```python
from build123d import *

# Parameters (mm, degrees)
F1_DEPTH    = 6.35
F4_T1_DEPTH = 6.35
F2_W        = 2.032
F2_H        = 2.032
F5_DEPTH    = 0.508
F7_R        = 0.1905
F12_DEPTH   = 0.254


# Not quite as in the source:
# - a fillet or chamfer that OpenCascade refuses, or shapes differently, is made with other operations: its cross-section is extruded or revolved along the edge and cut away or added


with BuildPart() as f1:
    # F0 (on Front) → F1 (new body)
    with BuildSketch(Plane.XZ):
        with BuildLine():
            Line((0, 0.7623671392), (0, 0))
            Line((0, 0), (9.652, 0))
            Line((9.652, 0), (9.652, 0.7623671392))
            Line((9.652, 0.7623671392), (6.0225553446, 1.5280881198))
            Line((6.0225553446, 1.5280881198), (6.0735776823, 1.729142969))
            Line((6.0735776823, 1.729142969), (5.8725685775, 1.7715508037))
            Line((5.8725685775, 1.7715508037), (5.8107842668, 1.5280881198))
            ThreePointArc((5.8107842668, 1.5280881198), (4.826, 0.762), (3.8412157332, 1.5280881198))
            Line((3.8412157332, 1.5280881198), (3.7794314225, 1.7715508037))
            Line((3.7794314225, 1.7715508037), (3.5784223177, 1.729142969))
            Line((3.5784223177, 1.729142969), (3.6294446554, 1.5280881198))
            Line((3.6294446554, 1.5280881198), (0, 0.7623671392))
        make_face()
    extrude(amount=-F1_DEPTH)

    # F4: fillet of radius 0.254 on 2 edges, made by hand

    # F4_s2 → F4_t1 (join)
    with BuildSketch(Plane.XZ.offset(-6.35)):
        with BuildLine():
            ThreePointArc((6.2750780534, 1.4748122183), (6.1284229129, 1.5656081597), (6.0735776823, 1.729142969))
            Line((6.0735776823, 1.729142969), (6.0225553446, 1.5280881198))
            Line((6.0225553446, 1.5280881198), (6.2750780534, 1.4748122183))
        make_face()
        with BuildLine():
            ThreePointArc((3.5784223177, 1.729142969), (3.5235770871, 1.5656081597), (3.3769219466, 1.4748122183))
            Line((3.3769219466, 1.4748122183), (3.6294446554, 1.5280881198))
            Line((3.6294446554, 1.5280881198), (3.5784223177, 1.729142969))
        make_face()
    extrude(amount=F4_T1_DEPTH)

    # F2 (on face) → F5 (join)
    with BuildSketch(Plane(origin=(0.5652924546, 0, 2.6794324958), x_dir=(0.9784612522, 0, -0.2064305646), z_dir=(0.2064305646, 0, 0.9784612522))):
        with Locations((7.3553929503, 3.175)):
            Rectangle(F2_W, F2_H)
    f5 = extrude(amount=F5_DEPTH)

    # F6: F5 across plane
    add(f5.mirror(Plane.YZ.offset(4.826)))

    # F7
    f7_edges = [f1.edges().sort_by_distance(p)[0] for p in [
        (9.652, 3.175, 0.762367),
        (0, 3.175, 0.762367),
        (7.963539, 6.35, 1.11859),
        (7.963539, 0, 1.11859),
        (1.688461, 0, 1.11859),
        (1.688461, 6.35, 1.11859),
        (9.652, 0, 0.381184),
        (9.652, 6.35, 0.381184),
        (0, 0, 0.381184),
        (0, 6.35, 0.381184),
        (3.523577, 6.35, 1.565608),
        (3.523577, 0, 1.565608),
        (6.128423, 0, 1.565608),
        (6.128423, 6.35, 1.565608),
    ]]
    fillet(f7_edges, radius=F7_R)


with BuildPart() as f8_1:
    # F8: copy of F1
    add(f1.part)


with BuildPart() as f9_1:
    # F9: copy of F8_1
    add(f8_1.part)


with BuildPart() as f1_1:
    add(f1.part)

    # F12 (add): a face of the model
    f12_faces = [f1_1.faces().sort_by_distance(p)[0] for p in [
        (4.826, 3.175, 0),
    ]]
    extrude(f12_faces, amount=F12_DEPTH)


solid = f1_1.part
```
The model under review builds one solid part; all positions refer to its coordinate system, in mm. A direction names the side the tool comes from. Round coordinates to 2 decimals unless told otherwise and drop trailing zeros. Order: outer loops, then holes, each group sorted by start corner. A loop starts at its lowest first (then second) coordinate and runs counter-clockwise, first axis right, second up. Notation, with made-up numbers: M 5.25,-17.5 L 19.25,-17.5 A26 cw 19.25,4.5 Z; hole C 45,54 d6. An arc over 180 degrees is marked long. Use a Markdown table: item, result.
1) Draft analysis for pull direction Z (two halves, no side actions). For faces 1 (the face through (9.652, 3, 0)), 2 (the face through (4.845, 3.131, 0.762)), 3 (the face through (5, 3, -0.254)), state which applies: released by +Z, released by -Z, zero draft, split by the parting line, or undercut.
Report:
| item | result |
|---|---|
| face 1 | zero draft |
| face 2 | released by +Z |
| face 3 | released by -Z |
2) Insertion check: pin 1 (1 mm diameter, centred on y = 2.5, z = 1.5, fed in from -X); pin 2 (0.5 mm diameter, centred on x = 8, z = 1.5, fed in from +Y); pin 3 (0.7 mm diameter, centred on x = 8, z = 1.5, fed in from -Y). Each pin has a flat end and moves straight along its axis. Give the tip position at first contact, or say it passes through.
Report:
| item | result |
|---|---|
| pin 1 | x = 0.79 |
| pin 2 | y = 4.19 |
| pin 3 | y = 2.16 |
3) Tool access review of faces 4 (the face through (7.8, 2.159, 1.4)), 5 (the face through (7.8, 4.191, 1.4)), 6 (the face through (1.9, 4.191, 1.4)), 7 (the face through (1.9, 2.159, 1.4)): name each direction out of +Z, -Z, +X, -X, +Y, -Y from which nothing blocks a thin tool from reaching the whole face with its end or side.
Report:
| item | result |
|---|---|
| face 4 | +Z, +X, -Y |
| face 5 | +Z, +X, +Y |
| face 6 | +Z, -X, +Y |
| face 7 | +Z, -X, -Y |
4) Wall thickness on line 1 along Y through (x, z) = (1.25, 1.5); line 2 along X through (y, z) = (5, 1.55); line 3 along Z through (x, y) = (2.5, 0.75): over which ranges is each line inside the solid? List them lowest first. Write a range as [from, to].
Report:
| item | result |
|---|---|
| line 1 | [2.16, 4.19] |
| line 2 | [3.51, 3.84], [5.82, 6.14] |
| line 3 | [-0.25, 1.29] |
5) Consider section C-C (x = 5.25). Write out the cut boundary in (y, z).
Report:
| item | result |
|---|---|
| outline | M 0,-0.25 L 6.35,-0.25 L 6.35,0.85 L 0,0.85 Z |
6) Consider section A-A (y = 5). Write out the cut boundary in (x, z), then the cut area to 3 significant figures.
Report:
| item | result |
|---|---|
| outline | M 0,-0.25 L 9.65,-0.25 L 9.65,0.61 A0.19 ccw 9.5,0.79 L 6.28,1.47 A0.25 cw 6.07,1.73 L 5.87,1.77 L 5.81,1.53 A1.02 cw 3.84,1.53 L 3.78,1.77 L 3.58,1.73 A0.25 cw 3.38,1.47 L 0.15,0.79 A0.19 ccw 0,0.61 Z |
| area | 13.4 mm^2 |
7) Consider section B-B (y = 3.5). Write out the cut boundary in (x, z), then the cut area to 3 significant figures.
Report:
| item | result |
|---|---|
| outline | M 0,-0.25 L 9.65,-0.25 L 9.65,0.61 A0.19 ccw 9.5,0.79 L 8.76,0.95 L 8.86,1.45 L 6.87,1.87 L 6.77,1.37 L 6.28,1.47 A0.25 cw 6.07,1.73 L 5.87,1.77 L 5.81,1.53 A1.02 cw 3.84,1.53 L 3.78,1.77 L 3.58,1.73 A0.25 cw 3.38,1.47 L 2.88,1.37 L 2.78,1.87 L 0.79,1.45 L 0.9,0.95 L 0.15,0.79 A0.19 ccw 0,0.61 Z |
| area | 15.5 mm^2 |
